Autodesk Inventor part; units mm, degrees
ref_plane "YZ Plane" through (0, 0, 0) normal (1, 0, 0) x (0, 1, 0)
ref_plane "XZ Plane" through (0, 0, 0) normal (0, 1, 0) x (-1, 0, 0)
ref_plane "XY Plane" through (0, 0, 0) normal (0, 0, 1) x (1, 0, 0)
sketch "Sketch1" plane through (0, 0, 0) normal (0, 1, 0) x (-1, 0, 0)
  line L0 (-15.0305, 11.0939) -> (8.4695, 11.0939)
  line L1 (8.4695, 11.0939) -> (8.4695, -12.4061)
  line L2 (8.4695, -12.4061) -> (6.9695, -12.4061)
  line L3 (6.9695, -12.4061) -> (6.9695, 9.5939)
  line L4 (6.9695, 9.5939) -> (-15.0305, 9.5939)
  line L5 (-15.0305, 9.5939) -> (-15.0305, 11.0939)
  point P0 (0, 0)
  dimension "d0" = 23.5
  dimension "d1" = 23.5
  dimension "d2" = 1.5
  dimension "d3" = 1.5
extrude "Extrusion1" add sketch "Sketch1" along normal blind 10
sketch "Sketch2" plane through (15.0305, 0, 9.5939) normal (0, 0, -1) x (-1, 0, 0)
  circle A0 centre (5, 5) radius 1.5
  circle A1 centre (17, 5) radius 1.5
  line L0 (0, 10) -> (22, 10)
  line L1 (0, 0) -> (0, 10)
  line L2 (23.5, 0) -> (23.5, 10)
  point P0 (15.0305, 0)
  dimension "d6" = 3
  dimension "d7" = 3
  dimension "d8" = 5
  dimension "d9" = 5
  dimension "d10" = 5
  dimension "d11" = 6.5
extrude "Extrusion2" cut sketch "Sketch2" against normal up to next
sketch "Sketch3" plane through (-6.9695, 0, 9.5939) normal (1, 0, 0) x (0, 0, -1)
  circle A0 centre (6.5, 5) radius 1.5
  line L0 (0, 10) -> (22, 10)
  line L1 (-1.5, 0) -> (-1.5, 10)
  point P0 (9.5939, 0)
  dimension "d14" = 3
  dimension "d15" = 5
  dimension "d16" = 8
extrude "Extrusion3" cut sketch "Sketch3" against normal up to next
properties part number "equerre_basse"
Read the model definition and answer for the solid it produces. Units are mm, in the model's axes. A direction names the side the tool comes from. Coordinates: 2 decimals unless noted, no trailing zeros. Write each loop counter-clockwise with the first axis right and the second up, starting at its lowest first coordinate (ties: lowest second). Pieces come first, ordered by that corner, then holes. Notation, with made-up numbers: (-11, 48) -> (46, 48) arc R31 cw to (46, 83) -> close; hole circle Ø7 at (12, -6). An arc over 180 degrees is marked (long way). Write item = value, one per line.
(1) Section D-D on y = 2 is taken. Write down the section's boundary in (x, z), plus the area to 4 significant figures.
From the geometry:
outline = (-8.47, -12.41) -> (-6.97, -12.41) -> (-6.97, 9.59) -> (15.03, 9.59) -> (15.03, 11.09) -> (-8.47, 11.09) -> close
area = 68.25 mm2
(2) Section A-A on y = 5 is taken. Write down the section's boundary in (x, z).
From the geometry:
outline = (-8.47, -12.41) -> (-6.97, -12.41) -> (-6.97, 1.59) -> (-8.47, 1.59) -> close; (-8.47, 4.59) -> (-6.97, 4.59) -> (-6.97, 9.59) -> (-3.47, 9.59) -> (-3.47, 11.09) -> (-8.47, 11.09) -> close; (-0.47, 9.59) -> (8.53, 9.59) -> (8.53, 11.09) -> (-0.47, 11.09) -> close; (11.53, 9.59) -> (15.03, 9.59) -> (15.03, 11.09) -> (11.53, 11.09) -> close
(3) Section C-C on z = 0 is taken. Write down the section's boundary in (x, y).
From the geometry:
outline = (-8.47, 0) -> (-6.97, 0) -> (-6.97, 10) -> (-8.47, 10) -> close
(4) Section B-B on x = 10 is taken. Write down the section's boundary in (y, z), plus the area to 3 significant figures.
From the geometry:
outline = (0, 9.59) -> (3.5, 9.59) -> (3.5, 11.09) -> (0, 11.09) -> close; (6.5, 9.59) -> (10, 9.59) -> (10, 11.09) -> (6.5, 11.09) -> close
area = 10.5 mm2
(5) Given pin 1 Ø6 at (x, y) = (6.5, 5.5) entering from -Z; pin 2 Ø3 at (y, z) = (7.5, -1) entering from +X, each flat-ended and moving along its own axis, determine where each tip first touches the part or whether it passes through.
From the geometry:
pin_1 = 9.59
pin_2 = -6.97
(6) Which of the six approach directions +Z, -Z, +X, -X, +Y, -Y give full straight-line access (tool end or side, diameter ignored) to faces 1 (the face through (-6.97, 5, -2)), 2 (the face through (15.03, 5, 10))?
From the geometry:
face_1 = -Z, +X, +Y, -Y
face_2 = +Z, -Z, +X, +Y, -Y
(7) For a pull along Y with two mould halves and no side action, classify faces 3 (the face through (8.645, 4.425, 10.333)), 4 (the face through (4, 5, 9.594)), 5 (the face through (-2, 10, 10)), 6 (the face through (-2, 0, 10)) as +Y half, -Y half, draft (parallel to the pull), parting line (faces both ways), or undercut.
From the geometry:
face_3 = undercut
face_4 = draft
face_5 = +Y half
face_6 = -Y half
(8) Straight lines are drawn through the part: L1, parallel to X at y = 9.75, z = -1; L2, parallel to Z at x = -2.75, y = 1; L3, parallel to X at y = 6, z = 10.25. For each, find the intervals that lie inside material, in ascending order. Write a range as from..to.
From the geometry:
L1 = -8.47..-6.97
L2 = 9.59..11.09
L3 = -8.47..-3.09, -0.85..8.91, 11.15..15.03
